Verification items for the finished model (mm, model axes). A direction names the side the tool comes from. Give positions to 0.01 mm unless a question says otherwise; leave off trailing zeros. Write each loop counter-clockwise with the first axis right and the second up, starting at its lowest first coordinate (ties: lowest second). Pieces come first, ordered by that corner, then holes.
Autodesk Inventor part; units mm, degrees
ref_plane "YZ Plane" through (0, 0, 0) normal (1, 0, 0) x (0, 1, 0)
ref_plane "XZ Plane" through (0, 0, 0) normal (0, 1, 0) x (-1, 0, 0)
ref_plane "XY Plane" through (0, 0, 0) normal (0, 0, 1) x (1, 0, 0)
sketch "Sketch3" plane through (0, 0, 0) normal (0, 0, 1) x (1, 0, 0)
  line L0 (0, 0) -> (6.25, 0)
  line L1 (6.25, 0) -> (6.25, -2)
  line L2 (1.5, 25) -> (7.5, 25)
  line L3 (7.5, 25) -> (7.5, 26.6)
  line L4 (10.5, 21) -> (10.5, -2)
  line L5 (6.25, -2) -> (10.5, -2)
  line L6 (7.5, 26.6) -> (9.5, 26.6)
  line L7 (9.5, 26.6) -> (9.5, 34.6)
  line L8 (9.5, 34.6) -> (10.5, 34.6)
  line L9 (10.5, 34.6) -> (10.5, 21)
  line L10 (1.5, 25) -> (1.5, 21)
  line L11 (1.5, 21) -> (0, 21)
  line L12 (0, 21) -> (0, 0)
  dimension "d5" = 4.25
  dimension "d7" = 1.6
  dimension "d10" = 1
  dimension "d13" = 2
  dimension "d16" = 3
  dimension "d17" = 8
  dimension "d18" = 25
  dimension "d19" = 1.5
  dimension "d20" = 4
  dimension "d21" = 10.5
  dimension "d23" = 6.25
revolve "Revolution1" add sketch "Sketch3" angle 360 about axis through (10.5, 21, 0) along (0, -1, 0)
fillet "Fillet1" radius 1.5 3 edges at (19.5, 25, 0) (21, 0, 0) (21, 21, 0)
sketch "Sketch4" plane through (10.5, 25, 0) normal (0, 1, 0) x (1, 0, 0)
  circle A0 centre (0, 0) radius 1
  circle A1 centre (0, 0) radius 5 construction
  circle A2 centre (-5, 0) radius 1.15
  line L0 (-14.7, 0) -> (14.7, 0)
  circle A3 centre (5, 0) radius 1.15
  point P0 (-10.5, 0)
  dimension "d24" = 10
  dimension "d25" = 2.3
  dimension "d28" = 360
extrude "Extrusion2" cut sketch "Sketch4" against normal blind 2 contours A2 L0 | L0 A2 | A3 L0 | L0 A3
sketch "Sketch6" plane through (10.5, 34.6, 0) normal (0, 1, 0) x (1, 0, 0)
  circle A0 centre (0, 0) radius 1
  point P0 (-10.5, 0)
extrude "Extrusion4" add sketch "Sketch6" along normal blind 1
properties part number "MOTOR"
Item 1: Set-up check for faces 4 (the face through (11.672, 22.233, -8.923)), 5 (the face through (0.5, 10.4, -3.2)): record each of +Z, -Z, +X, -X, +Y, -Y from which the full face is reachable in a straight line by a thin tool's end or side.
Answer key:
face 4: +Y
face 5: +Y, -Y
Item 2: Release check for a two-part mould opening along Z. For faces 1 (the face through (6.6, 0, -2.1)), 2 (the face through (8.215, -1.014, -3.584)), 3 (the face through (4.35, 24.01, -0.05)) record: released by +Z, released by -Z, zero draft, split by the parting line, or undercut.
Answer key:
face 1: zero draft
face 2: split by the parting line
face 3: undercut
Item 3: Sectioned sample at D-D on y = 20. Record the cut outline in (x, z).
Answer key:
outline: circle Ø20.83 at (10.5, 0)
Item 4: Depth check by flat-ended pin: pin 1 (1.2 mm diameter, centred on x = 6, z = -0.5, fed in from +Y); pin 2 (1 mm diameter, centred on x = 14.5, y = 22, fed in from -Z); pin 3 (5 mm diameter, centred on x = 5, z = -5, fed in from -Y). Enter the tip coordinate at first touch or a pass-through.
Answer key:
pin 1: stops at y = 25
pin 2: stops at z = -8.29
pin 3: stops at y = 0
Item 5: Scan lines: line 1 along X through (y, z) = (23.55, 0); line 2 along Y through (x, z) = (8, -2.25); line 3 along Z through (x, y) = (5.5, 24.4). Record each from-to range of solid material in increasing order.
Answer key:
line 1: x = 1.5 to 4.35, 6.65 to 14.35, 16.65 to 19.5
line 2: y = -2 to 25
line 3: z = -7.12 to -1.15, 1.15 to 7.12
Item 6: Sectioned sample at C-C on y = 6.5. Record the cut outline in (x, z).
Answer key:
outline: circle Ø21 at (10.5, 0)
